Could you check a few things on this model? Use its own coordinates, in mm. Round coordinates to 2 decimals unless told otherwise and drop trailing zeros. Loops run counter-clockwise (first coordinate to the right, second up) from the corner with the lowest first, then second, coordinate; pieces in that order, holes last. Notation, with made-up numbers: (-6, 30) - (21, 30) arc R37 ccw to (21, 67) - close; hole circle Ø9 at (-6.75, -1). An arc over 180 degrees is marked (long way). Use one line per item in the form item = value.
```python
from build123d import *

# Parameters (mm, degrees)
ESBO_O1_W                = 26
ESBO_O1_H                = 30
ESBO_O1_R                = 3.5
ESBO_O1_R_2              = 1.6
RESSALTO_EXTRUS_O1_DEPTH = 3
FILETE1_R                = 5


with BuildPart() as part:
    # Esboço1 → Ressalto-extrusão1 (new body)
    with BuildSketch(Plane.XY):
        Rectangle(ESBO_O1_W, ESBO_O1_H)
        Circle(ESBO_O1_R, mode=Mode.SUBTRACT)
        with Locations((8, 10)):
            Circle(ESBO_O1_R_2, mode=Mode.SUBTRACT)
        with Locations((-8, 10)):
            Circle(ESBO_O1_R_2, mode=Mode.SUBTRACT)
        with Locations((8, -10)):
            Circle(ESBO_O1_R_2, mode=Mode.SUBTRACT)
        with Locations((-8, -10)):
            Circle(ESBO_O1_R_2, mode=Mode.SUBTRACT)
    extrude(amount=RESSALTO_EXTRUS_O1_DEPTH)

    # Filete1
    filete1_edges = [part.edges().sort_by_distance(p)[0] for p in [
        (-13, -15, 1.5),
        (-13, 15, 1.5),
        (13, 15, 1.5),
        (13, -15, 1.5),
    ]]
    fillet(filete1_edges, radius=FILETE1_R)


solid = part.part
```
1. If we section it at C-C, the plane z = 2.15: Write out the boundary of the cut face in (x, y).
Solution:
outline = (-13, -10) arc R5 ccw to (-8, -15) - (8, -15) arc R5 ccw to (13, -10) - (13, 10) arc R5 ccw to (8, 15) - (-8, 15) arc R5 ccw to (-13, 10) - close; hole circle Ø3.2 at (-8, -10); hole circle Ø3.2 at (-8, 10); hole circle Ø7 at (0, 0); hole circle Ø3.2 at (8, -10); hole circle Ø3.2 at (8, 10)
2. If we section it at D-D, the plane x = 9.25: Write out the boundary of the cut face in (y, z), plus the area to 3 significant figures.
Solution:
outline = (-14.84, 0) - (-11, 0) - (-11, 3) - (-14.84, 3) - close; (-9, 0) - (9, 0) - (9, 3) - (-9, 3) - close; (11, 0) - (14.84, 0) - (14.84, 3) - (11, 3) - close
area = 77.1 mm^2
3. We'd pull the mould along X, two halves only. Please class faces 1 (the face through (3.233, -1.341, 1.479)), 2 (the face through (0, -15, 1)), 3 (the face through (-13, 0, 1)): +X half, -X half, draft (parallel to the pull), parting line (faces both ways), or undercut.
Solution:
face_1 = undercut
face_2 = draft
face_3 = -X half
4. If we section it at B-B, the plane x = 0: Write out the boundary of the cut face in (y, z), plus the area to 3 significant figures.
Solution:
outline = (-15, 0) - (-3.5, 0) - (-3.5, 3) - (-15, 3) - close; (3.5, 0) - (15, 0) - (15, 3) - (3.5, 3) - close
area = 69.0 mm^2
5. If we section it at A-A, the plane y = 0: Write out the boundary of the cut face in (x, z), plus the area to 3 significant figures.
Solution:
outline = (-13, 0) - (-3.5, 0) - (-3.5, 3) - (-13, 3) - close; (3.5, 0) - (13, 0) - (13, 3) - (3.5, 3) - close
area = 57.0 mm^2
6. Please list where these lines run through material, in increasing order: line 1 along Y through (x, z) = (8, 0.6); line 2 along Y through (x, z) = (-9, 0.2); line 3 along X through (y, z) = (-10.75, 1.1).
Solution:
line_1 = -15 to -11.6, -8.4 to 8.4, 11.6 to 15
line_2 = -14.9 to -11.25, -8.75 to 8.75, 11.25 to 14.9
line_3 = -12.94 to -9.41, -6.59 to 6.59, 9.41 to 12.94
7. For P1, Ø2.5, axis at x = 8, y = -10, coming from the +Z side, with a flat end and sliding along its axis, tell me the tip position at first contact or that it passes through.
Solution:
P1 = through
